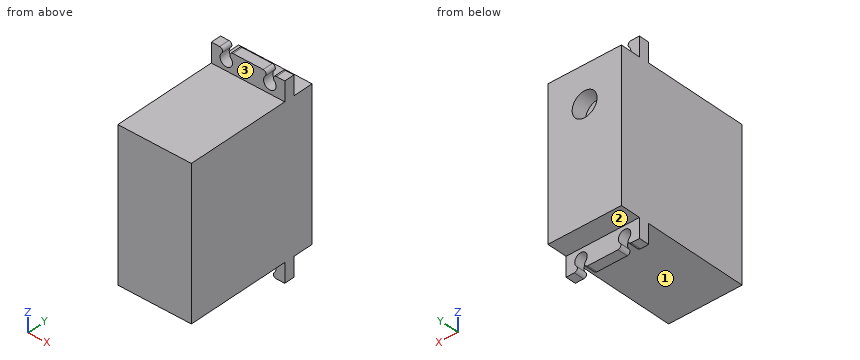
from build123d import *

# Parameters (mm, degrees)
SKETCH1_W           = 29.5
SKETCH1_H           = 59.5
BOSS_EXTRUDE1_DEPTH = 54.13
SKETCH2_W           = 29.5
SKETCH2_H           = 4.13
BOSS_EXTRUDE2_DEPTH = 7.75
CUT_EXTRUDE1_REACH  = 63.154
SKETCH4_R           = 5
CUT_EXTRUDE2_DEPTH  = 6


with BuildPart() as part:
    # Sketch1 → Boss-Extrude1 (new body)
    with BuildSketch(Plane(origin=(0, 0, 0), x_dir=(1, 0, 0), z_dir=(0, 1, 0))):
        Rectangle(SKETCH1_W, SKETCH1_H)
    extrude(amount=BOSS_EXTRUDE1_DEPTH)

    # Sketch2 → Boss-Extrude2 (add)
    with BuildSketch(Plane.XY.offset(29.75)):
        with Locations((0, 43.935)):
            Rectangle(SKETCH2_W, SKETCH2_H)
    boss_extrude2 = extrude(amount=BOSS_EXTRUDE2_DEPTH)

    # Sketch3 → Cut-Extrude1 (cut, up to next)
    with BuildSketch(Plane(origin=(0, 46, 0), x_dir=(1, 0, 0), z_dir=(0, 1, 0)), mode=Mode.PRIVATE) as cut_extrude1_sk1:
        with BuildLine():
            Line((6.079499649, -37.5), (11.375967158, -37.5))
            ThreePointArc((11.375967158, -37.5), (10.291171064, -36.779125945), (10.535567481, -35.49978535))
            ThreePointArc((10.535567481, -35.49978535), (8.765101817, -31.250045613), (6.943423266, -35.478085792))
            ThreePointArc((6.943423266, -35.478085792), (7.178874595, -36.774215218), (6.079499649, -37.5))
        make_face()
    cut_extrude1_tool1 = extrude(cut_extrude1_sk1.sketch, amount=-CUT_EXTRUDE1_REACH, mode=Mode.PRIVATE) & part.part
    # Sketch3 → Cut-Extrude1 (cut, up to next)
    with BuildSketch(Plane(origin=(0, 46, 0), x_dir=(1, 0, 0), z_dir=(0, 1, 0)), mode=Mode.PRIVATE) as cut_extrude1_sk2:
        with BuildLine():
            Line((-6.079499649, -37.5), (-11.375967158, -37.5))
            ThreePointArc((-11.375967158, -37.5), (-10.291171064, -36.779125945), (-10.535567481, -35.49978535))
            ThreePointArc((-10.535567481, -35.49978535), (-8.765101817, -31.250045613), (-6.943423266, -35.478085792))
            ThreePointArc((-6.943423266, -35.478085792), (-7.178874595, -36.774215218), (-6.079499649, -37.5))
        make_face()
    cut_extrude1_tool2 = extrude(cut_extrude1_sk2.sketch, amount=-CUT_EXTRUDE1_REACH, mode=Mode.PRIVATE) & part.part
    cut_extrude1_1 = cut_extrude1_tool1.solids().sort_by_distance((8.746301, 46, 34.352944))[0]
    add(cut_extrude1_1, mode=Mode.SUBTRACT)
    cut_extrude1_2 = cut_extrude1_tool2.solids().sort_by_distance((-8.746301, 46, 34.352944))[0]
    add(cut_extrude1_2, mode=Mode.SUBTRACT)
    cut_extrude1 = cut_extrude1_1 + cut_extrude1_2  # Cut-Extrude1 as one shape, for the pattern or mirror that repeats it

    # Mirror2: Boss-Extrude2, Cut-Extrude1 across plane
    add(boss_extrude2.mirror(Plane.XY))
    add(cut_extrude1.mirror(Plane.XY), mode=Mode.SUBTRACT)

    # Sketch4 → Cut-Extrude2 (cut)
    with BuildSketch(Plane(origin=(0, 54.13, 0), x_dir=(1, 0, 0), z_dir=(0, 1, 0))):
        with Locations(Location((0, -15, 0), (0, 0, 270))):
            Circle(SKETCH4_R)
    extrude(amount=-CUT_EXTRUDE2_DEPTH, mode=Mode.SUBTRACT)


solid = part.part
Design review of the part built by this model. Coordinates are the model's own, in mm. Face numbers are marked on the shaded views. A direction names the side the tool comes from. Coordinates: 2 decimals unless noted, no trailing zeros. Write each loop counter-clockwise with the first axis right and the second up, starting at its lowest first coordinate (ties: lowest second). Pieces come first, ordered by that corner, then holes. Notation, with made-up numbers: (-4, 70.25) -> (53, 70.25) arc R20 ccw to (53, 75.25) -> close; hole circle Ø7 at (67.25, 17). An arc over 180 degrees is marked (long way). Write each question's results on one line, items separated by ' | '. Start each with the question number.
(1) Tool access review of the marked faces 1, 2 and 3: name each direction out of +Z, -Z, +X, -X, +Y, -Y from which nothing blocks a thin tool from reaching the whole face with its end or side.
(2) For line 1 along X through (y, z) = (43.8, -33.75); line 2 along X through (y, z) = (43, 33); line 3 along Z through (x, y) = (3, 11), list the stretches that pass through material, from the lowest coordinate up. Write a range as from..to.
(3) Take a section at A-A on z = -33.75. Write out the cut boundary in (x, y).
(4) Take a section at C-C on z = 15. Write out the cut boundary in (x, y), and give its area (3 significant figures).
(5) Take a section at D-D on y = 16. Write out the cut boundary in (x, z).
(6) Clearance check with flat-ended pins moving along their axes: P1, Ø2.5, axis at x = 3, y = 52, coming from the +Z side; P2, Ø5, axis at x = 0.5, z = 13, coming from the +Y side; P3, Ø6.5, axis at x = 8.75, z = 33.75, coming from the -Y side; P4, Ø4, axis at x = -8.75, z = 33.75, coming from the +Y side. State where each tip first meets the part, or that it passes through.
(7) Take a section at B-B on x = 8.75. Write out the cut boundary in (y, z), and give its area (3 significant figures).
Results found:
1) face 1: -Z, +X, -X, -Y | face 2: -Z, +X, -X, +Y | face 3: +Z, +X, -X, -Y
2) line 1: x = -14.75..-11.25, -6.25..6.25, 11.25..14.75 | line 2: x = -14.75..-11.13, -6.37..6.37, 11.13..14.75 | line 3: z = -29.75..29.75
3) outline: (-14.75, 41.87) -> (-11.25, 41.87) -> (-11.25, 46) -> (-14.75, 46) -> close; (-6.25, 41.87) -> (6.25, 41.87) -> (6.25, 46) -> (-6.25, 46) -> close; (11.25, 41.87) -> (14.75, 41.87) -> (14.75, 46) -> (11.25, 46) -> close
4) outline: (-14.75, 0) -> (14.75, 0) -> (14.75, 54.13) -> (5, 54.13) -> (5, 48.13) -> (-5, 48.13) -> (-5, 54.13) -> (-14.75, 54.13) -> close | area: 1,540 mm2
5) outline: (-14.75, -29.75) -> (14.75, -29.75) -> (14.75, 29.75) -> (-14.75, 29.75) -> close
6) P1: stops at z = 29.75 | P2: stops at y = 48.13 | P3: stops at y = 41.87 | P4: passes through
7) outline: (0, -29.75) -> (41.87, -29.75) -> (41.87, -31.25) -> (46, -31.25) -> (46, -29.75) -> (54.13, -29.75) -> (54.13, 29.75) -> (46, 29.75) -> (46, 31.25) -> (41.87, 31.25) -> (41.87, 29.75) -> (0, 29.75) -> close | area: 3,230 mm2
